```python
from build123d import *

# Parameters (mm, degrees)
F0_R     = 6.858
F1_DEPTH = 1.27
F2_R     = 5.4864
F3_DEPTH = 6.35
F4_R     = 3.96875
F5_DEPTH = 25.4
F6_SIZE  = 0.79375
F7_R     = 0.396875


with BuildPart() as f1:
    # F0 (on Top) → F1 (new body)
    with BuildSketch(Plane.XY):
        Circle(F0_R)
    extrude(amount=F1_DEPTH)

    # F2 (on face) → F3 (join)
    with BuildSketch(Plane.XY.offset(1.27)):
        Circle(F2_R)
    extrude(amount=F3_DEPTH)

    # F4 (on Top) → F5 (cut)
    with BuildSketch(Plane.XY):
        Circle(F4_R)
    extrude(amount=F5_DEPTH, mode=Mode.SUBTRACT)

    # F6
    f6_edges = [f1.edges().sort_by_distance(p)[0] for p in [
        (-5.4864, 0, 7.62),
        (-3.96875, 0, 0),
    ]]
    chamfer(f6_edges, length=F6_SIZE)

    # F7
    f7_edges = [f1.edges().sort_by_distance(p)[0] for p in [
        (-6.858, 0, 0),
    ]]
    fillet(f7_edges, radius=F7_R)


solid = f1.part
```
The listing builds one solid part. Answer for the finished solid, in the listing's coordinates (mm). A direction names the side the tool comes from. Coordinates: 2 decimals unless noted, no trailing zeros. Loops run counter-clockwise (first coordinate to the right, second up) from the corner with the lowest first, then second, coordinate; pieces in that order, holes last. Notation, with made-up numbers: (53.25, 79.25) -> (66.25, 79.25) arc R23 cw to (66.25, 116.25) -> close; hole circle Ø1 at (74, -29). An arc over 180 degrees is marked (long way). Use one line per item in the form item = value. Start each with the question number.
Item 1: A tool of negligible diameter and unlimited length cuts with its end or side. For faces 1 (the face through (-3, 5, 1.27)), 2 (the face through (-4, 1, 7.62)), from which of +Z, -Z, +X, -X, +Y, -Y can it reach the whole face along a straight path? Write none if from no direction.
Item 2: The part is cut by section D-D on z = 7.25. Determine the outline of the cut face in (x, y), then the cut area to 3 significant figures.
Item 3: Consider L1, parallel to Z at x = -5.75, y = -3; L2, parallel to Y at x = 0, z = 5.75; L3, parallel to X at y = 1, z = 2. Determine where each line is inside the solid, lowest interval first. Write a range as [from, to].
Item 4: The part is cut by section A-A on x = 0. Determine the outline of the cut face in (y, z).
Item 5: The part is cut by section C-C on z = 1.5. Determine the outline of the cut face in (x, y), then the cut area to 3 significant figures.
Item 6: The mould has two halves that part along X. Classify faces 3 (the face through (-1, -5, 0)), 4 (the face through (-0.86, -3.874, 4.159)), 5 (the face through (-1.189, -5.356, 4.009)): released by +X, released by -X, zero draft, split by the parting line, or undercut.
Item 7: Flat-ended cylindrical pins translate along their axes: pin 1 Ø1 at (x, z) = (3, 2.5) entering from -Y; pin 2 Ø1 at (x, z) = (-2, 2) entering from -Y; pin 3 Ø7 at (x, y) = (0, 0) entering from +Z; pin 4 Ø6 at (x, y) = (1, 1) entering from -Z. Find the tip coordinate at first contact, or state that the pin passes through.
Answer key:
q1.face_1 = +Z
q1.face_2 = +Z, +X, -X, +Y, -Y
q2.outline = circle Ø10.13 at (0, 0); hole circle Ø7.94 at (0, 0)
q2.area = 31.0 mm2
q3.L1 = [0, 1.27]
q3.L2 = [-5.49, -3.97], [3.97, 5.49]
q3.L3 = [-5.39, -3.84], [3.84, 5.39]
q4.outline = (-6.86, 0.4) arc R0.4 ccw to (-6.46, 0) -> (-4.76, 0) -> (-3.97, 0.79) -> (-3.97, 7.62) -> (-4.69, 7.62) -> (-5.49, 6.83) -> (-5.49, 1.27) -> (-6.86, 1.27) -> close; (3.97, 0.79) -> (4.76, 0) -> (6.46, 0) arc R0.4 ccw to (6.86, 0.4) -> (6.86, 1.27) -> (5.49, 1.27) -> (5.49, 6.83) -> (4.69, 7.62) -> (3.97, 7.62) -> close
q5.outline = circle Ø10.97 at (0, 0); hole circle Ø7.94 at (0, 0)
q5.area = 45.1 mm2
q6.face_3 = zero draft
q6.face_4 = undercut
q6.face_5 = split by the parting line
q7.pin_1 = -4.88
q7.pin_2 = -5.28
q7.pin_3 = through
q7.pin_4 = 0.35
